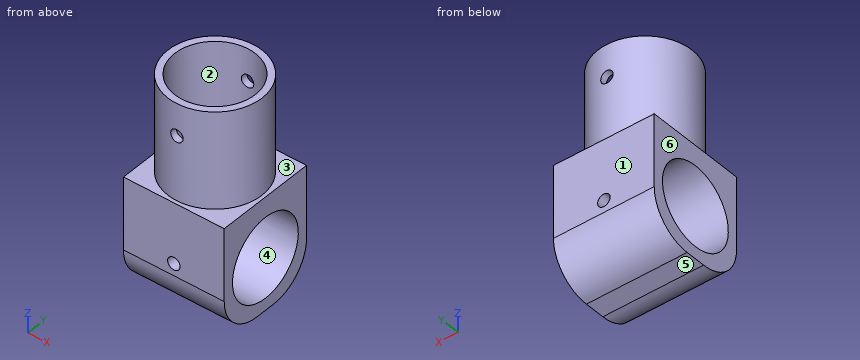
from build123d import *

# Parameters (mm, degrees)
SKETCH_1_W                  = 25
SKETCH_1_H                  = 28
EXTRUDE_1_DEPTH             = 25
SKETCH_2_W                  = 11.657397777
SKETCH_2_H                  = 24
HOLE_WIZARD_20_0_20_1_D     = 20
HOLE_WIZARD_20_0_20_2_D     = 20
HOLE_WIZARD_20_0_20_2_DEPTH = 23
FILLET_1_R                  = 10
CUT_EXTRUDE_1_DEPTH         = 35.766927543
CUT_EXTRUDE_1_DEPTH_BACK    = 35.766927543
SKETCH_7_R                  = 1.55
SKETCH_9_R                  = 1.55
CUT_EXTRUDE_2_DEPTH         = 41.957163608


with BuildPart() as part:
    # 草图1 → 凸台-拉伸1 (new body)
    with BuildSketch(Plane.XZ.offset(5.250668647)):
        with Locations((3.885641605, -14)):
            Rectangle(SKETCH_1_W, SKETCH_1_H)
    extrude(amount=-EXTRUDE_1_DEPTH)

    # 草图2 → 旋转1 (revolve)
    with BuildSketch(Plane.XZ.offset(-7.249331353), mode=Mode.PRIVATE) as revolve_1_sk:
        with Locations((9.714340494, 12)):
            Rectangle(SKETCH_2_W, SKETCH_2_H)
    revolve(revolve_1_sk.sketch.rotate(Axis((3.885641605, 7.249331353, 24), (0, 0, -1)), 180), axis=Axis((3.885641605, 7.249331353, 24), (0, 0, -1)))

    # Ø20.0 (20) 直径孔1 (through all)
    with Locations(Plane.ZY.offset(8.614358395)):
        with Locations((-15, 7.249331353)):
            Hole(HOLE_WIZARD_20_0_20_1_D / 2)

    # Ø20.0 (20) 直径孔2
    with Locations(Plane.XY.offset(24)):
        with Locations((3.885641605, 7.249331353)):
            Hole(HOLE_WIZARD_20_0_20_2_D / 2, depth=HOLE_WIZARD_20_0_20_2_DEPTH)

    # 圆角1
    fillet_1_edges = [part.edges().sort_by_distance(p)[0] for p in [
        (3.885641605, 19.749331353, -28),
        (3.885641605, -5.250668647, -28),
    ]]
    fillet(fillet_1_edges, radius=FILLET_1_R)

    # 草图7 → 切除-拉伸1 (cut, two sides: drawn at the far end of the back side and taken through both)
    with BuildSketch(Plane.XZ.offset(-7.249331353).offset(-CUT_EXTRUDE_1_DEPTH_BACK)):
        with Locations(Location((3.885641605, 16, 0), (0, 0, 270))):
            Circle(SKETCH_7_R)
    extrude(amount=CUT_EXTRUDE_1_DEPTH + CUT_EXTRUDE_1_DEPTH_BACK, mode=Mode.SUBTRACT)

    # 草图9 → 切除-拉伸2 (cut, through all)
    with BuildSketch(Plane(origin=(0, 19.749331353, 0), x_dir=(1, 0, 0), z_dir=(0, 1, 0))):
        with Locations(Location((3.885641605, 15, 0), (0, 0, 270))):
            Circle(SKETCH_9_R)
    extrude(amount=-CUT_EXTRUDE_2_DEPTH, mode=Mode.SUBTRACT)


solid = part.part
Could you check a few things on this model? Use its own coordinates, in mm. Face numbers are marked on the shaded views. A direction names the side the tool comes from. Coordinates: 2 decimals unless noted, no trailing zeros. Write each loop counter-clockwise with the first axis right and the second up, starting at its lowest first coordinate (ties: lowest second). Pieces come first, ordered by that corner, then holes. Notation, with made-up numbers: M -15,23 L 20,23 A14 cw 20,44 Z; hole C -22,61.25 d7. An arc over 180 degrees is marked long. One line per question, with ' | ' between items.
1) For pin 1 Ø1.5 at (x, z) = (13, -21.5) entering from -Y; pin 2 Ø8 at (x, y) = (9, -0.5) entering from -Z; pin 3 Ø5 at (x, z) = (10, 8) entering from +Y, each with a flat end and sliding along its axis, tell me the tip position at first contact or that it passes through.
Checks:
pin 1: y = -4.87 | pin 2: z = -27.92 | pin 3: y = 18.33
2) Imagine slicing it at C-C, the plane x = 10.5. Write out the boundary of the cut face in (y, z).
Checks:
outline: M -5.25,-18 A10 ccw 4.75,-28 L 9.75,-28 A10 ccw 19.75,-18 L 19.75,0 L 16.85,0 L 16.85,24 L 14.75,24 L 14.75,1 L -0.25,1 L -0.25,24 L -2.35,24 L -2.35,0 L -5.25,0 Z; hole C 7.25,-15 d20
3) Imagine slicing it at A-A, the plane z = -15. Write out the boundary of the cut face in (x, y).
Checks:
outline: M -8.61,-5.25 L 2.34,-5.25 L 2.34,-2.75 L -8.61,-2.75 Z; M -8.61,17.25 L 2.34,17.25 L 2.34,19.75 L -8.61,19.75 Z; M 5.44,-5.25 L 16.39,-5.25 L 16.39,-2.75 L 5.44,-2.75 Z; M 5.44,17.25 L 16.39,17.25 L 16.39,19.75 L 5.44,19.75 Z
4) For the marked faces 1 and 2, which set-ups out of +Z, -Z, +X, -X, +Y, -Y let a thin tool reach every point of the face, with its end or its side?
Checks:
face 1: +Z, -Z, +X, -X, +Y | face 2: +Z
5) Imagine slicing it at D-D, the plane y = 16.5. Write out the boundary of the cut face in (x, z), and give its area (3 significant figures).
Checks:
outline: M -8.61,-25.38 L 16.39,-25.38 L 16.39,-18.8 L -8.61,-18.8 Z; M -8.61,-11.2 L 16.39,-11.2 L 16.39,0 L 10.98,0 L 10.98,24 L 7.68,24 L 7.68,1 L 0.09,1 L 0.09,24 L -3.21,24 L -3.21,0 L -8.61,0 Z | area: 610 mm²
6) I need wall thicknesses on probe 1 along X at (y, z) = (19, -15); probe 2 along Z at (x, y) = (1, 8.75); probe 3 along Y at (x, z) = (7, -13). Which ranges of each line are inside material? Lowest first, please. Write a range as [from, to].
Checks:
probe 1: [-8.61, 2.34], [5.44, 16.39] | probe 2: [-28, -24.89], [-5.11, 1] | probe 3: [-5.25, -2.55], [17.05, 19.75]
7) If we mould it in two halves opening along Z, with no side actions, what happens to the marked faces 3, 4, 5 and 6? For each: released by +Z, released by -Z, zero draft, split by the parting line, or undercut.
Checks:
face 3: released by +Z | face 4: undercut | face 5: released by -Z | face 6: zero draft
